Build history of the part. All positions in model axes, mm. A direction names the side the tool comes from. Give positions to 0.01 mm unless a question says otherwise; leave off trailing zeros. Loops run counter-clockwise (first coordinate to the right, second up) from the corner with the lowest first, then second, coordinate; pieces in that order, holes last. Notation, with made-up numbers: (87, 30) -> (127, 30) arc R19 ccw to (127, 36) -> close; hole circle Ø4 at (26, 82.25). An arc over 180 degrees is marked (long way). One line per question, with ' | ' between items. Start each with the question number.
(1) Slice it at A-A, the plane z = 9. Give the number of separate pieces and of enclosed holes in the cut face, then the cut area to 3 significant figures.
(2) Drill centre lines: L1, parallel to X at y = -22.5, z = 9; L2, parallel to X at y = 3, z = 9; L3, parallel to Y at x = 0, z = -2. Where is each one in solid material? Low to high. Write a range as from..to.
(3) Slice it at C-C, the plane x = 0. Write the cut outline in (y, z).
(4) Slice it at B-B, the plane y = -5. Write the cut outline in (x, z), then the cut area to 3 significant figures.
(5) Slice it at D-D, the plane x = -34. Write the cut outline in (y, z), then the cut area to 3 significant figures.
(6) Mould opens along Z. For faces 1 (the face through (1, -22, -17.5)), 2 (the face through (-25.297, 5.334, 16.882)), 3 (the face through (-37, 1.42, 10)) say: pulls with the +Z half, pulls with the -Z half, needs draft (parallel to the pull), parting line crosses it, or undercut.
(7) Flat gauge pins, fed straight in: pin 1 Ø13.5 at (x, z) = (34, -7) entering from +Y; pin 2 Ø5 at (x, z) = (-34, 9) entering from -Y; pin 3 Ø3.5 at (y, z) = (14.5, 0.5) entering from -X; pin 4 Ø9 at (x, z) = (-34, -9) entering from +Y. Where does each tip first touch, or does it go through?
(8) 3-axis set-ups, long thin cutter, end or side, ignore diameter. For faces 4 (the face through (-3.6, 9.3, -6.5)), 5 (the face through (38.136, 3.235, -13.511)), 6 (the face through (-34, 5, 0)): which of +Z, -Z, +X, -X, +Y, -Y reach the whole face in a straight line?
```python
from build123d import *

# Parameters (mm, degrees)
SKETCH1_R                               = 16
BOSS_EXTRUDE1_DEPTH                     = 17.5
SKETCH2_R                               = 16
SKETCH2_R_2                             = 14.5
BOSS_EXTRUDE2_DEPTH                     = 6.5
SKETCH3_R                               = 2.6
CUT_EXTRUDE1_DEPTH                      = 58.771100041
CBORE_FOR_M5_HEX_HEAD_BOLT1_D           = 5.5
CBORE_FOR_M5_HEX_HEAD_BOLT1_CBORE_D     = 12.24
CBORE_FOR_M5_HEX_HEAD_BOLT1_CBORE_DEPTH = 3.58
CHAMFER1_SIZE                           = 2
FILLET1_R                               = 2
CHAMFER2_SIZE                           = 1


with BuildPart() as part:
    # Sketch1 → Boss-Extrude1 (new, symmetric)
    with BuildSketch(Plane.XY):
        Polygon((-25, -30), (-42.5, -30), (-42.5, 5), (-25, 5), (-25, 20), (25, 20), (25, 5), (42.5, 5), (42.5, -30), (25, -30), align=None)
        with Locations((0, -5)):
            Circle(SKETCH1_R, mode=Mode.SUBTRACT)
    extrude(amount=BOSS_EXTRUDE1_DEPTH, both=True)

    # Sketch2 → Boss-Extrude2 (add, symmetric)
    with BuildSketch(Plane.XY):
        with Locations((0, -5)):
            Circle(SKETCH2_R)
        with Locations(Location((0, -5, 0), (0, 0, 180))):
            Circle(SKETCH2_R_2, mode=Mode.SUBTRACT)
    extrude(amount=BOSS_EXTRUDE2_DEPTH, both=True)

    # Sketch3 → Cut-Extrude1 (cut, through all)
    with BuildSketch(Plane(origin=(0, 5, 0), x_dir=(1, 0, 0), z_dir=(0, 1, 0))):
        with Locations(Location((-34, 9, 0), (0, 0, 270))):
            Circle(SKETCH3_R)
        with Locations(Location((-34, -9, 0), (0, 0, 90))):
            Circle(SKETCH3_R)
        with Locations(Location((34, 9, 0), (0, 0, 90))):
            Circle(SKETCH3_R)
        with Locations(Location((34, -9, 0), (0, 0, 270))):
            Circle(SKETCH3_R)
    extrude(amount=-CUT_EXTRUDE1_DEPTH, mode=Mode.SUBTRACT)

    # CBORE for M5 Hex Head Bolt1 (through all)
    with Locations(Plane(origin=(-34, 5, -9), x_dir=(0, 0, 1), z_dir=(0, 1, 0))):
        with Locations((0, 0), (18, 0), (18, 68), (0, 68)):
            CounterBoreHole(CBORE_FOR_M5_HEX_HEAD_BOLT1_D / 2, CBORE_FOR_M5_HEX_HEAD_BOLT1_CBORE_D / 2, CBORE_FOR_M5_HEX_HEAD_BOLT1_CBORE_DEPTH)

    # Chamfer1
    chamfer1_edges = [part.edges().sort_by_distance(p)[0] for p in [
        (0, 20, -17.5),
        (-25, 20, 0),
        (25, 20, 0),
        (0, 20, 17.5),
    ]]
    chamfer(chamfer1_edges, length=CHAMFER1_SIZE)

    # Fillet1
    fillet1_edges = [part.edges().sort_by_distance(p)[0] for p in [
        (42.5, -12.5, -17.5),
        (-42.5, -12.5, 17.5),
        (-42.5, -12.5, -17.5),
        (25, 5, 0),
        (-25, 5, 0),
        (42.5, -12.5, 17.5),
    ]]
    fillet(fillet1_edges, radius=FILLET1_R)

    # Chamfer2
    chamfer2_edges = [part.edges().sort_by_distance(p)[0] for p in [
        (-33.75, 5, -17.5),
        (-42.5, 5, 0),
        (-33.75, 5, 17.5),
        (-41.914213562, 5, -16.914213562),
        (-41.914213562, 5, 16.914213562),
        (25, 12.5, 17.5),
        (33.75, 5, 17.5),
        (25, 12.5, -17.5),
        (33.75, 5, -17.5),
        (42.5, 5, 0),
        (41.914213562, 5, -16.914213562),
        (41.914213562, 5, 16.914213562),
        (-25.585786438, 5.585786438, -17.5),
        (-25.585786438, 5.585786438, 17.5),
        (25.585786438, 5.585786438, -17.5),
        (25.585786438, 5.585786438, 17.5),
        (-25, 12.5, 17.5),
        (-25, 12.5, -17.5),
    ]]
    chamfer(chamfer2_edges, length=CHAMFER2_SIZE)


solid = part.part
```
Final values:
1) separate pieces: 3 | enclosed holes: 1 | area: 2,480 mm2
2) L1: -42.5..-36.75, -31.25..31.25, 36.75..42.5 | L2: -42.5..-40.12, -27.88..-13.86, 13.86..27.88, 40.12..42.5 | L3: -30..-19.5, 9.5..20
3) outline: (-30, -17.5) -> (-21, -17.5) -> (-21, -6.5) -> (-19.5, -6.5) -> (-19.5, 6.5) -> (-21, 6.5) -> (-21, 17.5) -> (-30, 17.5) -> close; (9.5, -6.5) -> (11, -6.5) -> (11, -17.5) -> (18, -17.5) -> (20, -15.5) -> (20, 15.5) -> (18, 17.5) -> (11, 17.5) -> (11, 6.5) -> (9.5, 6.5) -> close
4) outline: (-42.5, -15.5) arc R2 ccw to (-40.5, -17.5) -> (-16, -17.5) -> (-16, -6.5) -> (-14.5, -6.5) -> (-14.5, 6.5) -> (-16, 6.5) -> (-16, 17.5) -> (-40.5, 17.5) arc R2 ccw to (-42.5, 15.5) -> close; (14.5, -6.5) -> (16, -6.5) -> (16, -17.5) -> (40.5, -17.5) arc R2 ccw to (42.5, -15.5) -> (42.5, 15.5) arc R2 ccw to (40.5, 17.5) -> (16, 17.5) -> (16, 6.5) -> (14.5, 6.5) -> close; hole circle Ø5.5 at (-34, -9); hole circle Ø5.5 at (-34, 9); hole circle Ø5.5 at (34, -9); hole circle Ø5.5 at (34, 9) | area: 1,800 mm2
5) outline: (-30, -17.5) -> (4, -17.5) -> (5, -16.5) -> (5, -15.12) -> (1.42, -15.12) -> (1.42, -11.75) -> (-30, -11.75) -> close; (-30, -6.25) -> (1.42, -6.25) -> (1.42, -2.88) -> (5, -2.88) -> (5, 2.88) -> (1.42, 2.88) -> (1.42, 6.25) -> (-30, 6.25) -> close; (-30, 11.75) -> (1.42, 11.75) -> (1.42, 15.12) -> (5, 15.12) -> (5, 16.5) -> (4, 17.5) -> (-30, 17.5) -> close | area: 791 mm2
6) face 1: pulls with the -Z half | face 2: pulls with the +Z half | face 3: undercut
7) pin 1: y = 5 | pin 2: through | pin 3: x = -25 | pin 4: y = 1.42
8) face 4: -Z | face 5: +Y | face 6: +Z, -Z, -X, +Y
